```python
from build123d import *

# Parameters (mm, degrees)
F1_DEPTH    = 14
F4_DEPTH    = 25
F7_DEPTH    = 25
F8_T1_DEPTH = 14
F9_T1_DEPTH = 14


# Not quite as in the source:
# - a fillet or chamfer that OpenCascade refuses, or shapes differently, is made with other operations: its cross-section is extruded or revolved along the edge and cut away or added


with BuildPart() as f1:
    # F0 (on Front) → F1 (new body)
    with BuildSketch(Plane.XZ):
        Polygon((-16.5, 2), (-27, 2), (-27, 0), (0, 0), (0, 2), (-7.5, 2), (-12, 2), align=None)
        Polygon((-12, 9), (-16.5, 2), (-12, 2), align=None)
        Polygon((-12, 9), (-12, 2), (-7.5, 2), align=None)
    extrude(amount=F1_DEPTH)

    # F3 (on face) → F4 (cut)
    with BuildSketch(Plane.XY.offset(9)):
        with BuildLine():
            ThreePointArc((-10.9640486734, -10), (-11.2569418922, -9.2928932188), (-11.9640486734, -9))
            Line((-11.9640486734, -9), (-11.9640486734, -10))
            Line((-11.9640486734, -10), (-11.9640486734, -11))
            ThreePointArc((-11.9640486734, -11), (-11.2569418922, -10.7071067812), (-10.9640486734, -10))
        make_face()
        with BuildLine():
            Line((-11.9640486734, -10), (-11.9640486734, -9))
            ThreePointArc((-11.9640486734, -9), (-12.9640486734, -10), (-11.9640486734, -11))
            Line((-11.9640486734, -11), (-11.9640486734, -10))
        make_face()
    extrude(amount=-F4_DEPTH, mode=Mode.SUBTRACT)

    # F6 (on offset) → F7 (cut)
    with BuildSketch(Plane.XZ.offset(14)):
        with BuildLine():
            Line((-11.884468704, 9.0000648052), (-12.0001798496, 9.0000648052))
            Line((-12.0001798496, 9.0000648052), (-12.253829136, 9.0000648052))
            ThreePointArc((-12.253829136, 9.0000648052), (-12.2044720661, 8.2484912646), (-12.0572486618, 7.5098274869))
            ThreePointArc((-12.0572486618, 7.5098274869), (-11.9278078867, 8.2499547835), (-11.884468704, 9.0000648052))
        make_face()
        with BuildLine():
            Line((-12.253829136, 9.0000648052), (-12.0001798496, 9.0000648052))
            Line((-12.0001798496, 9.0000648052), (-11.884468704, 9.0000648052))
            ThreePointArc((-11.884468704, 9.0000648052), (-11.9278078867, 9.7501748268), (-12.0572486618, 10.4903021234))
            ThreePointArc((-12.0572486618, 10.4903021234), (-12.2044720661, 9.7516383457), (-12.253829136, 9.0000648052))
        make_face()
        with BuildLine():
            ThreePointArc((-12.0572486618, 7.5098274869), (-12.2044720661, 8.2484912646), (-12.253829136, 9.0000648052))
            ThreePointArc((-12.253829136, 9.0000648052), (-12.2044720661, 9.7516383457), (-12.0572486618, 10.4903021234))
            ThreePointArc((-12.0572486618, 10.4903021234), (-24.9106333558, 9.0000648052), (-12.0572486618, 7.5098274869))
        make_face()
        with BuildLine():
            ThreePointArc((-12.0572486618, 10.4903021234), (-11.9278078867, 9.7501748268), (-11.884468704, 9.0000648052))
            ThreePointArc((-11.884468704, 9.0000648052), (-11.9278078867, 8.2499547835), (-12.0572486618, 7.5098274869))
            ThreePointArc((-12.0572486618, 7.5098274869), (-5.7553696033, 3.3025358829), (-0.7600571518, 9.0000648052))
            ThreePointArc((-0.7600571518, 9.0000648052), (-5.7553696033, 14.6975937274), (-12.0572486618, 10.4903021234))
        make_face()
    extrude(amount=-F7_DEPTH, mode=Mode.SUBTRACT)

    # F8: fillet of radius 5 on 1 edges, made by hand

    # F8_s2 → F8_t1 (join)
    with BuildSketch(Plane.XZ):
        with BuildLine():
            ThreePointArc((-18.8598420152, 2), (-17.2756076516, 2.2576164768), (-15.854623238, 3.0039194075))
            Line((-15.854623238, 3.0039194075), (-16.5, 2))
            Line((-16.5, 2), (-18.8598420152, 2))
        make_face()
    extrude(amount=F8_T1_DEPTH)

    # F9: fillet of radius 5 on 1 edges, made by hand

    # F9_s2 → F9_t1 (join)
    with BuildSketch(Plane.XZ):
        with BuildLine():
            ThreePointArc((-8.5459751266, 3.6270724192), (-6.8718408683, 2.4248148724), (-4.8549915809, 2))
            Line((-4.8549915809, 2), (-7.5, 2))
            Line((-7.5, 2), (-8.5459751266, 3.6270724192))
        make_face()
    extrude(amount=F9_T1_DEPTH)


solid = f1.part
```
CAD build for the part. Positions are in the model's coordinates, mm. A direction names the side the tool comes from. Round coordinates to 2 decimals unless told otherwise and drop trailing zeros. Loops run counter-clockwise (first coordinate to the right, second up) from the corner with the lowest first, then second, coordinate; pieces in that order, holes last. Notation, with made-up numbers: M 66,27 L 114,27 A4 cw 114,34 Z; hole C 38.5,26 d3. An arc over 180 degrees is marked long. Use a Markdown table: item, result. Add a question column.
(1) Cut at B-B (z = 4.5). Give the cut face in (x, y).
(2) Which spindle directions (+Z, -Z, +X, -X, +Y, -Y) get a long thin tool onto all of the face, cutting with end or side? Do faces 1 (the face through (-23, -7, 2)), 2 (the face through (-2, -7, 2)), 3 (the face through (-12, 0, 2)). Say none if no direction does.
(3) Cut at A-A (y = -2). Give the cut face in (x, z) (3 decimals).
(4) Cut at C-C (z = 2.5). Give the cut face in (x, y).
(5) Flat gauge pin, fed straight in: pin 1 (6.5 mm diameter, centred on x = -21.5, y = -9.5, fed in from +Z). Where does the tip first touch, or does it go through?
(6) Drill centre lines: line 1 (Z direction, x = -2, y = -2.5); line 2 (X direction, y = -10.5, z = 4.5); line 3 (Y direction, x = -11.5, z = 4.5). Where is each one in solid material? Low to high.
Geometry says:
| question | item | result |
|---|---|---|
| 1 | outline | M -13.69,-14 L -10.08,-14 L -10.08,0 L -13.69,0 Z; hole C -11.96,-10 d2 |
| 2 | face 1 | +Z, -X, +Y, -Y |
| 2 | face 2 | +Z, +X, +Y, -Y |
| 2 | face 3 | +Z, -Z, +X, -X, +Y |
| 3 | outline | M -27,0 L 0,0 L 0,2 L -4.855,2 A5 cw -8.546,3.627 A5.747 cw -12.057,7.51 A6.513 cw -15.855,3.004 A5 cw -18.86,2 L -27,2 Z |
| 4 | outline | M -16.68,-14 L -7.03,-14 L -7.03,0 L -16.68,0 Z; hole C -11.96,-10 d2 |
| 5 | pin 1 | stops at z = 2.04 |
| 6 | line 1 | z = 0 to 2 |
| 6 | line 2 | x = -13.69 to -12.83, -11.1 to -10.08 |
| 6 | line 3 | y = -14 to -10.89, -9.11 to 0 |
